Verification items for the finished model (mm, model axes). A direction names the side the tool comes from. Give positions to 0.01 mm unless a question says otherwise; leave off trailing zeros. Loops run counter-clockwise (first coordinate to the right, second up) from the corner with the lowest first, then second, coordinate; pieces in that order, holes last. Notation, with made-up numbers: (-14.75, 6.25) - (13.25, 6.25) arc R19 ccw to (13.25, 35.25) - close; hole circle Ø6 at (24.25, 72.5). An arc over 180 degrees is marked (long way). One line per item, written item: value. Start each with the question number.
1. Access from +Z, -Z, +X, -X, +Y, -Y to the whole of each face (thin tool, end or side, straight path). Record for faces 4 (the flat face through (87, -29, -19.05)), 5 (the flat face through (75, -25, -25.4)).
2. Sectioned sample at D-D (y = -15). Count the separate pieces of the cut face and the enclosed holes in it, plus the area to 3 significant figures.
3. Sectioned sample at C-C (z = 55). Record the cut outline in (x, y), plus the area to 3 significant figures.
4. Mould release check, pull along X, two halves, no side actions. Record for faces 1 (the flat face through (23.6, -50.8, 8.4)), 2 (the flat face through (90, -6.35, 24)), 3 (the cylindrical face through (42.363, -25.044, 66.547)): pulls with the +X half, pulls with the -X half, needs draft (parallel to the pull), parting line crosses it, or undercut.
5. Sectioned sample at B-B (x = 79). Record the cut outline in (y, z), plus the area to 3 significant figures.
6. Gauge pin test, flat ends, axial feed: pin 1 (8 mm diameter, centred on x = 75.5, y = -12, fed in from +Z); pin 2 (3 mm diameter, centred on y = -35.5, z = 16, fed in from -X); pin 3 (17 mm diameter, centred on x = 0, z = 0, fed in from -Y); pin 4 (1.5 mm diameter, centred on x = 105, y = -39, fed in from +Z). Record the tip position at first contact, or that the pin passes through.
7. Sectioned sample at A-A (z = 7.5). Record the cut outline in (x, y), plus the area to 3 significant figures.
8. Scan lines: L1, parallel to X at y = -23.5, z = -2; L2, parallel to Y at x = 27, z = -9.5; L3, parallel to Z at x = 29, y = -19.5. Record each from-to range of solid material in increasing order. Write a range as [from, to].
from build123d import *

# Parameters (mm, degrees)
F1_DEPTH = 50.8
F3_DEPTH = 44.45
F4_R     = 9.525
F5_DEPTH = 50.801
F6_R     = 6.35


with BuildPart() as f1:
    # F0 (on Front) → F1 (new body)
    with BuildSketch(Plane.XZ):
        with BuildLine():
            ThreePointArc((-18.842481, 17.032936), (9.125815, 23.703998), (25.4, 0))
            ThreePointArc((25.4, 0), (17.960512, -17.960512), (0, -25.4))
            Line((0, -25.4), (152.4, -25.4))
            Line((152.4, -25.4), (152.4, 63.5))
            ThreePointArc((152.4, 63.5), (100.824266, 38.70075), (113.659667, 94.470918))
            ThreePointArc((113.659667, 94.470918), (41.420002, 65.998851), (-18.842481, 17.032936))
        make_face()
        with BuildLine():
            ThreePointArc((152.4, 63.5), (140.475734, 88.29925), (113.659667, 94.470918))
            ThreePointArc((113.659667, 94.470918), (100.824266, 38.70075), (152.4, 63.5))
        make_face()
        with BuildLine():
            ThreePointArc((0, -25.4), (17.960512, -17.960512), (25.4, 0))
            ThreePointArc((25.4, 0), (9.125815, 23.703998), (-18.842481, 17.032936))
            ThreePointArc((-18.842481, 17.032936), (-23.214183, -10.308332), (0, -25.4))
        make_face()
    extrude(amount=F1_DEPTH)

    # F2 (on face) → F3 (cut)
    with BuildSketch(Plane.XZ.offset(50.8)):
        with BuildLine():
            ThreePointArc((115.057734, 88.276734), (52.250613, 64.79482), (-1.954932, 25.324657))
            ThreePointArc((-1.954932, 25.324657), (17.255503, 18.638874), (25.4, 0))
            ThreePointArc((25.4, 0), (23.150521, -10.450521), (16.800521, -19.05))
            Line((16.800521, -19.05), (146.05, -19.05))
            Line((146.05, -19.05), (146.05, 63.5))
            ThreePointArc((146.05, 63.5), (136.510587, 83.3394), (115.057734, 88.276734))
        make_face()
    extrude(amount=-F3_DEPTH, mode=Mode.SUBTRACT)

    # F4 (on face) → F5 (cut, through all)
    with BuildSketch(Plane.XZ.offset(50.8)):
        Circle(F4_R)
    extrude(amount=-F5_DEPTH, mode=Mode.SUBTRACT)

    # F6
    f6_edges = [f1.edges().sort_by_distance(p)[0] for p in [
        (16.800521, -28.575, -19.05),
        (-1.954932, -28.575, 25.324657),
    ]]
    fillet(f6_edges, radius=F6_R)


solid = f1.part
Results are:
1. face 4: -Y
1. face 5: -Z, +X, -X, +Y, -Y
2. separate pieces: 1
2. enclosed holes: 2
2. area: 4,450 mm^2
3. outline: (24.23, -50.8) - (35.63, -50.8) - (35.63, -6.35) - (146.05, -6.35) - (146.05, -50.8) - (152.4, -50.8) - (152.4, 0) - (24.23, 0) - close
3. area: 1,600 mm^2
4. face 1: needs draft
4. face 2: undercut
4. face 3: pulls with the -X half
5. outline: (-50.8, -25.4) - (0, -25.4) - (0, 84) - (-50.8, 84) - (-50.8, 77.19) - (-6.35, 77.19) - (-6.35, -19.05) - (-50.8, -19.05) - close
5. area: 1,280 mm^2
6. pin 1: stops at z = 84.19
6. pin 2: stops at x = -20.85
6. pin 3: passes through
6. pin 4: stops at z = 92.55
7. outline: (-24.27, -50.8) - (-5.87, -50.8) - (-5.87, 0) - (-24.27, 0) - close; (5.87, -50.8) - (24.27, -50.8) - (24.27, -6.35) - (146.05, -6.35) - (146.05, -50.8) - (152.4, -50.8) - (152.4, 0) - (5.87, 0) - close
7. area: 2,960 mm^2
8. L1: x = [-25.32, -9.31], [9.31, 25.32], [146.05, 152.4]
8. L2: y = [-6.35, 0]
8. L3: z = [-25.4, -19.05], [50.58, 58.25]
